Input: dimensioned drawing with shaded views. Units: mm. Origin: part minimum x, y, z. A direction names the side the tool comes from. Coordinates: 2 decimals unless noted, no trailing zeros. Write each loop counter-clockwise with the first axis right and the second up, starting at its lowest first coordinate (ties: lowest second). Pieces come first, ordered by that corner, then holes. Notation, with made-up numbers: M 15.5,89.5 L 69.5,89.5 A15 cw 69.5,100.5 Z; hole C 42,48 d7. An arc over 180 degrees is marked long. Use one line per item in the form item = value.
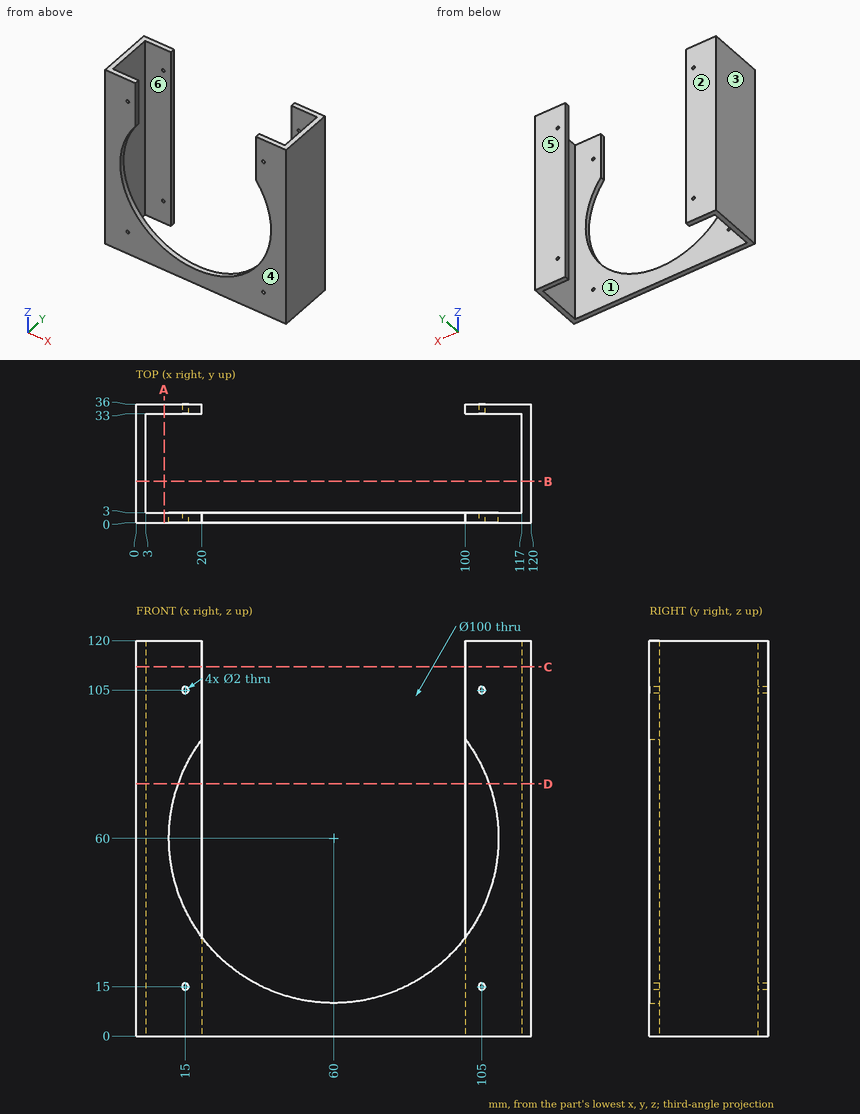
(1) Section query B-B on y = 12.5. Return the cut outline in (x, z), plus the area to 3 significant figures.
Computed:
outline = M 0,0 L 3,0 L 3,120 L 0,120 Z; M 117,0 L 120,0 L 120,120 L 117,120 Z
area = 720 mm^2
(2) Line query: probe 1 along X at (y, z) = (2.35, 105); probe 2 along X at (y, z) = (6.5, 82); probe 3 along Z at (x, y) = (15, 1.9). Output: solid intervals per line, ascending.
Computed:
probe_1 = 0 to 14, 16 to 20, 100 to 104, 106 to 120
probe_2 = 0 to 3, 117 to 120
probe_3 = 0 to 14, 16 to 38.21, 81.79 to 104, 106 to 120
(3) Section query C-C on z = 112. Return the cut outline in (x, y), plus the area to 3 significant figures.
Computed:
outline = M 0,0 L 20,0 L 20,3 L 3,3 L 3,33 L 20,33 L 20,36 L 0,36 Z; M 100,0 L 120,0 L 120,36 L 100,36 L 100,33 L 117,33 L 117,3 L 100,3 Z
area = 420 mm^2
(4) Set-up query: the marked faces 1 and 2. Return all of +Z, -Z, +X, -X, +Y, -Y with unobstructed straight access to the full face (end or side cutting, diameter ignored); none if empty.
Computed:
face_1 = +Z, -Z
face_2 = +Z, -Z, +X, -X, +Y
(5) Section query D-D on z = 76.5. Return the cut outline in (x, y).
Computed:
outline = M 0,0 L 12.8,0 L 12.8,3 L 3,3 L 3,33 L 20,33 L 20,36 L 0,36 Z; M 100,33 L 117,33 L 117,3 L 107.2,3 L 107.2,0 L 120,0 L 120,36 L 100,36 Z
(6) Pull-direction query (Y, two-part tool) for the marked faces 3, 4, 5 and 6; classes: pulls with the +Y half, pulls with the -Y half, needs draft (parallel to the pull), parting line crosses it, or undercut.
Computed:
face_3 = needs draft
face_4 = pulls with the -Y half
face_5 = pulls with the +Y half
face_6 = undercut
(7) Section query A-A on x = 8.5. Return the cut outline in (y, z).
Computed:
outline = M 0,0 L 3,0 L 3,120 L 0,120 Z; M 33,0 L 36,0 L 36,120 L 33,120 Z
